from build123d import *

# Parameters (mm, degrees)
SKETCH_R  = 2.5
PAD_DEPTH = 300
FILLET_R  = 1.5


with BuildPart() as part:
    # Sketch → Pad (new body)
    with BuildSketch(Plane.XY):
        Polygon((-3.6, 2.53934), (-3.6, -2.53934), (-6.56066, -5.5), (-7.9, -5.5), (-7.9, -3.1), (-9.5, -3.1), (-10, -3.6), (-10, -10), (-3.6, -10), (-3.1, -9.5), (-3.1, -7.9), (-5.5, -7.9), (-5.5, -6.56066), (-2.53934, -3.6), (2.53934, -3.6), (5.5, -6.56066), (5.5, -7.9), (3.1, -7.9), (3.1, -9.5), (3.6, -10), (10, -10), (10, -3.6), (9.5, -3.1), (7.9, -3.1), (7.9, -5.5), (6.56066, -5.5), (3.6, -2.53934), (3.6, 2.53934), (6.56066, 5.5), (7.899992, 5.5), (7.899998, 3.1), (9.5, 3.1), (10, 3.6), (10, 10), (3.6, 10), (3.1, 9.5), (3.1, 7.9), (5.5, 7.9), (5.5, 6.56066), (2.53934, 3.6), (-2.53934, 3.6), (-5.5, 6.56066), (-5.5, 7.9), (-3.1, 7.9), (-3.1, 9.5), (-3.6, 10), (-10, 10), (-10, 3.6), (-9.5, 3.1), (-7.9, 3.1), (-7.9, 5.5), (-6.56066, 5.5), align=None)
        Circle(SKETCH_R, mode=Mode.SUBTRACT)
    extrude(amount=PAD_DEPTH)

    # Fillet
    fillet_edges = [part.edges().sort_by_distance(p)[0] for p in [
        (-10, -10, 150),
        (10, -10, 150),
        (10, 10, 150),
        (-10, 10, 150),
    ]]
    fillet(fillet_edges, radius=FILLET_R)


solid = part.part
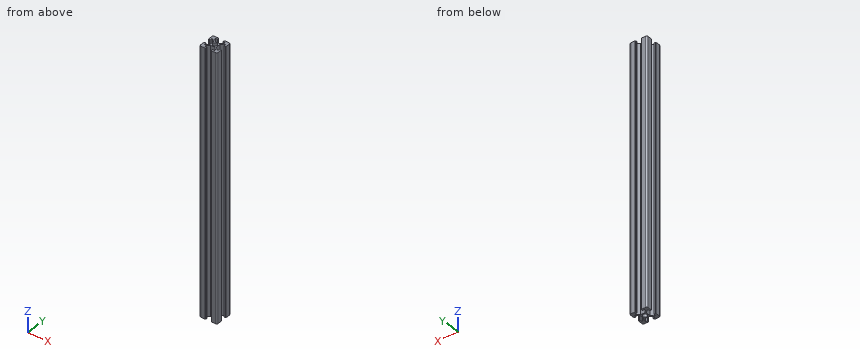
Here's how the part is built. I have some questions about the finished solid (model axes, mm). Coordinates: 2 decimals unless noted, no trailing zeros. Order: outer loops, then holes, each group sorted by start corner. A loop starts at its lowest first (then second) coordinate and runs counter-clockwise, first axis right, second up.
Item 1: If we section it at A-A on y = 0: List the corners of the cut face in (x, z) for me.
Result sheet:
outline: (-3.6, 0) - (-2.5, 0) - (-2.5, 300) - (-3.6, 300) - close; (2.5, 0) - (3.6, 0) - (3.6, 300) - (2.5, 300) - close
Item 2: I need wall thicknesses on line 1 (Y direction, x = 0, z = 196); line 2 (Y direction, x = 4.5, z = 242); line 3 (X direction, y = 7, z = 176). Which ranges of each line are inside material? Lowest first, please.
Result sheet:
line 1: y = -3.6 to -2.5, 2.5 to 3.6
line 2: y = -10 to -7.9, -5.56 to -3.44, 3.44 to 5.56, 7.9 to 10
line 3: x = -10 to -5.5, 5.5 to 10
Item 3: For P1, Ø1.5, axis at y = 0.5, z = 138.5, coming from the +X side; P2, Ø2, axis at y = -2.5, z = 169, coming from the +X side; P3, Ø3, axis at x = 0, y = 0, coming from the +Z side; P4, Ø2, axis at y = 0, z = 94.5, coming from the -X side, each with a flat end and sliding along its axis, tell me the tip position at first contact or that it passes through.
Result sheet:
P1: stops at x = 3.6
P2: stops at x = 9.9
P3: passes through
P4: stops at x = -3.6
